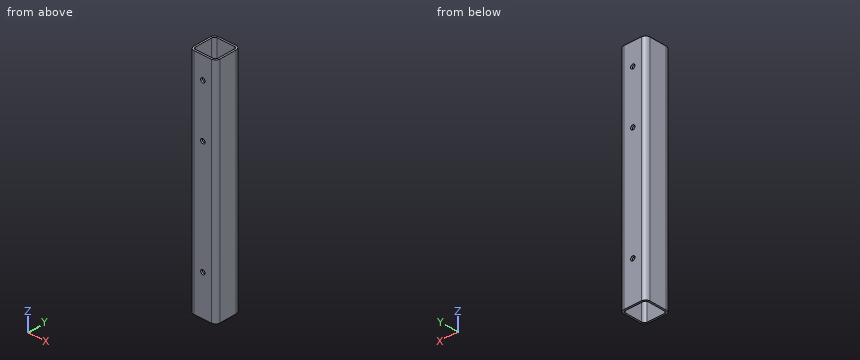
from build123d import *

# Parameters (mm, degrees)
AUFSATZ_LINEAR_AUSTRAGEN1_DEPTH = 130
SKIZZE2_R                       = 2.5
SCHNITT_LINEAR_AUSTRAGEN1_DEPTH = 60


with BuildPart() as part:
    # Skizze1 → Aufsatz-Linear austragen1 (new, symmetric)
    with BuildSketch(Plane.XY):
        with BuildLine():
            Line((-10, 15), (10, 15))
            ThreePointArc((10, 15), (13.535533906, 13.535533906), (15, 10))
            Line((15, 10), (15, -10))
            ThreePointArc((15, -10), (13.535533906, -13.535533906), (10, -15))
            Line((10, -15), (-10, -15))
            ThreePointArc((-10, -15), (-13.535533906, -13.535533906), (-15, -10))
            Line((-15, -10), (-15, 10))
            ThreePointArc((-15, 10), (-13.535533906, 13.535533906), (-10, 15))
        make_face()
        with BuildLine():
            Line((-13, 10), (-13, -10))
            ThreePointArc((-13, -10), (-12.121320344, -12.121320344), (-10, -13))
            Line((-10, -13), (10, -13))
            ThreePointArc((10, -13), (12.121320344, -12.121320344), (13, -10))
            Line((13, -10), (13, 10))
            ThreePointArc((13, 10), (12.121320344, 12.121320344), (10, 13))
            Line((10, 13), (-10, 13))
            ThreePointArc((-10, 13), (-12.121320344, 12.121320344), (-13, 10))
        make_face(mode=Mode.SUBTRACT)
    extrude(amount=AUFSATZ_LINEAR_AUSTRAGEN1_DEPTH, both=True)

    # Skizze2 → Schnitt-Linear austragen1 (cut)
    with BuildSketch(Plane.XZ.offset(15)):
        with Locations(Location((0, -84, 0), (0, 0, 270))):
            Circle(SKIZZE2_R)
        with Locations(Location((0, 105, 0), (0, 0, 270))):
            Circle(SKIZZE2_R)
        with Locations(Location((0, 45, 0), (0, 0, 270))):
            Circle(SKIZZE2_R)
    extrude(amount=-SCHNITT_LINEAR_AUSTRAGEN1_DEPTH, mode=Mode.SUBTRACT)


solid = part.part
Design review of the part built by this model. Coordinates are the model's own, in mm. Coordinates: 2 decimals unless noted, no trailing zeros. Order: outer loops, then holes, each group sorted by start corner. A loop starts at its lowest first (then second) coordinate and runs counter-clockwise, first axis right, second up.
Item 1: Take a section at B-B, the plane z = -84. Write out the cut boundary in (x, y), then the cut area to 3 significant figures.
Item 2: Take a section at D-D, the plane z = 71.5. Write out the cut boundary in (x, y), then the cut area to 3 significant figures.
Item 3: For line 1 (X direction, y = -1.5, z = 27.5); line 2 (X direction, y = 11.25, z = 0), list the stretches that pass through material, from the lowest coordinate up.
Item 4: For pin 1 Ø12 at (x, y) = (4, 0) entering from -Z, flat-tipped, find the tip position at first contact; note if it passes through.
Item 5: Take a section at A-A, the plane x = 0. Count the separate pieces of the cut face and the enclosed holes in it, then the cut area to 3 significant figures.
Item 6: Take a section at C-C, the plane y = -6.5. Write out the cut boundary in (x, z), then the cut area to 3 significant figures.
The answers:
1. outline: (-15, -10) arc R5 ccw to (-10, -15) - (-2.5, -15) - (-2.5, -13) - (-10, -13) arc R3 cw to (-13, -10) - (-13, 10) arc R3 cw to (-10, 13) - (-2.5, 13) - (-2.5, 15) - (-10, 15) arc R5 ccw to (-15, 10) - close; (2.5, -15) - (10, -15) arc R5 ccw to (15, -10) - (15, 10) arc R5 ccw to (10, 15) - (2.5, 15) - (2.5, 13) - (10, 13) arc R3 cw to (13, 10) - (13, -10) arc R3 cw to (10, -13) - (2.5, -13) - close
1. area: 190 mm2
2. outline: (-15, -10) arc R5 ccw to (-10, -15) - (10, -15) arc R5 ccw to (15, -10) - (15, 10) arc R5 ccw to (10, 15) - (-10, 15) arc R5 ccw to (-15, 10) - close; hole (-13, -10) arc R3 ccw to (-10, -13) - (10, -13) arc R3 ccw to (13, -10) - (13, 10) arc R3 ccw to (10, 13) - (-10, 13) arc R3 ccw to (-13, 10) - close
2. area: 210 mm2
3. line 1: x = -15 to -13, 13 to 15
3. line 2: x = -14.84 to -12.73, 12.73 to 14.84
4. pin 1: passes through
5. separate pieces: 8
5. enclosed holes: 0
5. area: 980 mm2
6. outline: (-15, -130) - (-13, -130) - (-13, 130) - (-15, 130) - close; (13, -130) - (15, -130) - (15, 130) - (13, 130) - close
6. area: 1,040 mm2
